Could you check a few things on this model? Use its own coordinates, in mm. Face numbers are marked on the shaded views. A direction names the side the tool comes from. Round coordinates to 2 decimals unless told otherwise and drop trailing zeros. Loops run counter-clockwise (first coordinate to the right, second up) from the corner with the lowest first, then second, coordinate; pieces in that order, holes last.
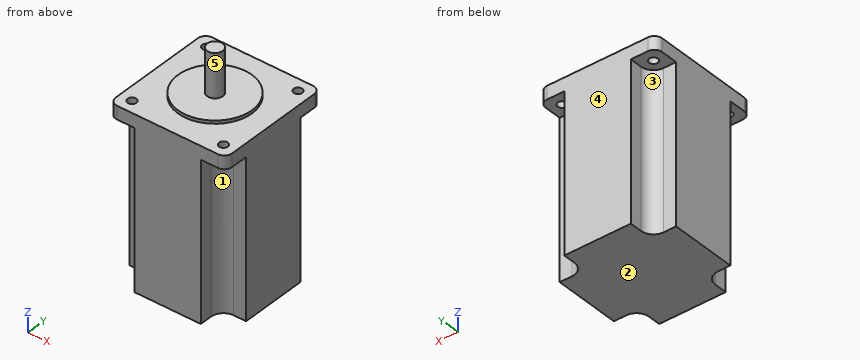
Autodesk Inventor part; units mm, degrees
ref_plane "YZ Plane" through (0, 0, 0) normal (1, 0, 0) x (0, 1, 0)
ref_plane "XZ Plane" through (0, 0, 0) normal (0, 1, 0) x (-1, 0, 0)
ref_plane "XY Plane" through (0, 0, 0) normal (0, 0, 1) x (1, 0, 0)
sketch "Skizze1" plane through (0, 0, 0) normal (0, 0, 1) x (1, 0, 0)
  line L0 (-26, -30) -> (26, -30)
  line L1 (30, -26) -> (30, 26)
  line L2 (26, 30) -> (-26, 30)
  line L3 (-30, 26) -> (-30, -26)
  line L4 (-30, -30) -> (30, 30) construction
  line L5 (30, -30) -> (-30, 30) construction
  arc A0 (30, 26) -> (26, 30) centre (26, 26) ccw
  arc A1 (26, -30) -> (30, -26) centre (26, -26) ccw
  arc A2 (-30, -26) -> (-26, -30) centre (-26, -26) ccw
  arc A3 (-26, 30) -> (-30, 26) centre (-26, 26) ccw
  point P0 (0, 0)
  dimension "d0" = 4
  dimension "d1" = 60
extrude "Extrusion1" add sketch "Skizze1" against normal blind 88
sketch "Skizze2" plane through (0, 0, 0) normal (0, 0, 1) x (1, 0, 0)
  circle A0 centre (0, 0) radius 19.05
  dimension "d4" = 38.1
extrude "Extrusion2" add sketch "Skizze2" along normal blind 1.6
sketch "Skizze4" plane through (0, 0, 0) normal (0, 0, 1) x (1, 0, 0)
  circle A0 centre (0, 0) radius 19.05
  line L0 (30, 26) -> (30, -26)
  arc A1 (30, 26) -> (26, 30) centre (26, 26) ccw
  line L1 (-26, 30) -> (26, 30)
  arc A2 (-26, 30) -> (-30, 26) centre (-26, 26) ccw
  line L2 (-30, -26) -> (-30, 26)
  arc A3 (-30, -26) -> (-26, -30) centre (-26, -26) ccw
  line L3 (26, -30) -> (-26, -30)
  arc A4 (26, -30) -> (30, -26) centre (26, -26) ccw
  line L4 (26, -26) -> (-26, 26) construction
  line L5 (-23.57, 23.57) -> (23.57, 23.57) construction
  line L6 (23.57, 23.57) -> (23.57, -23.57) construction
  line L7 (23.57, -23.57) -> (-23.57, -23.57) construction
  line L8 (-23.57, -23.57) -> (-23.57, 23.57) construction
  line L9 (-23.57, 23.57) -> (23.57, -23.57) construction
  line L10 (23.57, 23.57) -> (-23.57, -23.57) construction
  dimension "d15" = 47.14
hole "Bohrung1" at (23.57, 23.57, 0) at (-23.57, 23.57, 0) at (-23.57, -23.57, 0) at (23.57, -23.57, 0) direction (0, 0, -1) diameter 4.5 end through all
sketch "Skizze5" plane through (0, 0, 1.6) normal (0, 0, 1) x (1, 0, 0)
  circle A0 centre (0, 0) radius 4
  dimension "d23" = 8
extrude "Extrusion4" add sketch "Skizze5" along normal blind 22.4
sketch "Skizze7" plane through (0, 0, -88) normal (0, 0, -1) x (-1, 0, 0)
  circle A0 centre (23.57, -23.57) radius 2.25
  circle A1 centre (-23.57, 23.57) radius 2.25
  circle A2 centre (23.57, 23.57) radius 2.25
  circle A3 centre (-23.57, -23.57) radius 2.25
  line L0 (-30, 26) -> (-30, -26)
  arc A4 (-30, -26) -> (-26, -30) centre (-26, -26) ccw
  line L1 (-26, -30) -> (26, -30)
  arc A5 (26, -30) -> (30, -26) centre (26, -26) ccw
  line L2 (30, -26) -> (30, 26)
  arc A6 (30, 26) -> (26, 30) centre (26, 26) ccw
  line L3 (26, 30) -> (-26, 30)
  arc A7 (-26, 30) -> (-30, 26) centre (-26, 26) ccw
  circle A8 centre (23.57, -23.57) radius 6.43 construction
  line L4 (30, -26) -> (30, 26)
  line L5 (30, -17.14) -> (23.57, -17.14)
  line L6 (-26, -30) -> (26, -30)
  line L7 (17.14, -30) -> (17.14, -23.57)
  arc A9 (23.57, -17.14) -> (17.14, -23.57) centre (23.57, -23.57) ccw
  arc A10 (-17.14, -23.57) -> (-23.57, -17.14) centre (-23.57, -23.57) ccw
  arc A11 (17.2019, 24.4599) -> (23.57, 17.14) centre (23.57, 23.57) ccw
  arc A12 (-23.57, 17.14) -> (-17.14, 23.57) centre (-23.57, 23.57) ccw
  line L8 (23.57, 17.14) -> (30, 17.14)
  line L9 (17.14, 23.57) -> (17.14, 30)
  line L10 (26, 30) -> (-26, 30)
  line L11 (-17.14, 23.57) -> (-17.14, 30)
  line L12 (-23.57, 17.14) -> (-30, 17.14)
  line L13 (-23.57, -17.14) -> (-30, -17.14)
  line L14 (-17.14, -23.57) -> (-17.14, -30)
  point P0 (0, 0)
extrude "Extrusion6" cut sketch "Skizze7" against normal blind 81.2 contours A7 L3 L11 A12 L12 L0 | L13 A10 L14 L1 A4 L0 | L3 A6 L2 L8 A11 L9 | L7 A9 L5 L2 A5 L1
sketch "Skizze8" plane through (0, 0, -88) normal (0, 0, -1) x (-1, 0, 0)
  circle A0 centre (23.57, -23.57) radius 2.25 construction
  circle A1 centre (-23.57, 23.57) radius 2.25 construction
  circle A2 centre (23.57, 23.57) radius 2.25 construction
  circle A3 centre (-23.57, -23.57) radius 2.25 construction
  circle A4 centre (0, 0) radius 19.05 construction
  line L0 (-30, 26) -> (-30, -26) construction
  arc A5 (-26, 30) -> (-30, 26) centre (-26, 26) ccw construction
  line L1 (26, 30) -> (-26, 30) construction
  arc A6 (30, 26) -> (26, 30) centre (26, 26) ccw construction
  line L2 (30, -26) -> (30, 26) construction
  arc A7 (26, -30) -> (30, -26) centre (26, -26) ccw construction
  line L3 (-26, -30) -> (26, -30) construction
  arc A8 (-30, -26) -> (-26, -30) centre (-26, -26) ccw construction
  circle A9 centre (0, 0) radius 42.4264 construction
  line L4 (30, 30) -> (-30, 30) construction
  line L5 (-30, 30) -> (-30, -30) construction
  line L6 (-30, -30) -> (30, -30) construction
  line L7 (30, -30) -> (30, 30) construction
  line L8 (30, 30) -> (-30, -30) construction
  line L9 (-30, 30) -> (30, -30) construction
  line L10 (-17.14, -30) -> (17.14, -30) construction
  line L11 (-30, 17.14) -> (-30, -17.14) construction
equation "\"d1\" = breite"
equation "\"d2\" = Laenge"
equation "\"d4\" = fit"
equation "\"d5\" = fit_l"
equation "\"d15\" = lochabstand"
equation "\"d16\" = bohrung_d"
equation "\"d23\" = schaft_d"
equation "\"d24\" = schaft_l"
equation "\"d28\" = Laenge - Mount_l"
equation "\"breite\" = 60"
equation "\"lochabstand\" = 47.14"
equation "\"schaft_d\" = 8"
equation "\"fit\" = 38.1"
equation "\"fit_l\" = 1.6"
equation "\"Mount_l\" = 6.8"
equation "\"Laenge\" = 88"
equation "\"bohrung_d\" = 4.5"
properties part number "Nema24"
Item 1: If we section it at B-B, the plane y = 7: Please give me the cut outline in (x, z).
Results list:
outline: (-30, -88) - (30, -88) - (30, 0) - (17.72, 0) - (17.72, 1.6) - (-17.72, 1.6) - (-17.72, 0) - (-30, 0) - close
Item 2: If we section it at C-C, the plane z = -20: Please give me the cut outline in (x, y).
Results list:
outline: (-30, -17.14) - (-23.57, -17.14) arc R6.43 cw to (-17.14, -23.57) - (-17.14, -30) - (17.14, -30) - (17.14, -23.57) arc R6.43 cw to (23.57, -17.14) - (30, -17.14) - (30, 17.14) - (23.57, 17.14) arc R6.43 cw to (17.14, 23.57) - (17.14, 30) - (-17.14, 30) - (-17.14, 23.57) arc R6.43 cw to (-23.57, 17.14) - (-30, 17.14) - close
Item 3: Will these pins go through, and if not, where does the flat tip stop? pin 1 (5 mm diameter, centred on y = 27, z = -45, fed in from +X); pin 2 (1.9 mm diameter, centred on x = -27.5, z = -35.5, fed in from +Y); pin 3 (3 mm diameter, centred on y = -27.5, z = -50.5, fed in from -X).
Results list:
pin 1: stops at x = 17.14
pin 2: stops at y = 17.14
pin 3: stops at x = -17.14
Item 4: If we section it at A-A, the plane x = 0: Please give me the cut outline in (y, z), then the cut area to 3 significant figures.
Results list:
outline: (-30, -88) - (30, -88) - (30, 0) - (19.05, 0) - (19.05, 1.6) - (4, 1.6) - (4, 24) - (-4, 24) - (-4, 1.6) - (-19.05, 1.6) - (-19.05, 0) - (-30, 0) - close
area: 5,520 mm2
Item 5: For the marked faces 1, 2, 3, 4 and 5, which set-ups out of +Z, -Z, +X, -X, +Y, -Y let a thin tool reach every point of the face, with its end or its side?
Results list:
face 1: -Z, +X, -Y
face 2: -Z, +X, -X, +Y, -Y
face 3: -Z, -X, +Y
face 4: +Z, -Z, +X, -X, +Y
face 5: +Z
Item 6: If we section it at D-D, the plane x = 15.5: Please give me the cut outline in (y, z).
Results list:
outline: (-30, -88) - (30, -88) - (30, 0) - (11.07, 0) - (11.07, 1.6) - (-11.07, 1.6) - (-11.07, 0) - (-30, 0) - close
Item 7: If I drill on line 1 along Y through (x, z) = (-23.57, -4.5); line 2 along Y through (x, z) = (23, -5), over which ranges is the centre line in solid material (lowest first)?
Results list:
line 1: y = -30 to -25.82, -21.32 to 21.32, 25.82 to 30
line 2: y = -30 to -25.75, -21.39 to 21.39, 25.75 to 30
